Geometry: final body of the model. Coordinates: model frame, mm. A direction names the side the tool comes from. Coordinates: 2 decimals unless noted, no trailing zeros. Order: outer loops, then holes, each group sorted by start corner. A loop starts at its lowest first (then second) coordinate and runs counter-clockwise, first axis right, second up. Notation, with made-up numbers: M -20,84 L -2,84 A28 cw -2,107 Z; hole C -17,76 d5. An arc over 180 degrees is marked long. One line per question, with ' | ' between items.
Autodesk Inventor part; units mm, degrees
ref_plane "YZ Plane" through (0, 0, 0) normal (1, 0, 0) x (0, 1, 0)
ref_plane "XZ Plane" through (0, 0, 0) normal (0, 1, 0) x (-1, 0, 0)
ref_plane "XY Plane" through (0, 0, 0) normal (0, 0, 1) x (1, 0, 0)
sketch "Boceto1" plane through (0, 0, 0) normal (0, 1, 0) x (-1, 0, 0)
  line L0 (-14.8958, 23.7803) -> (7.8042, 23.7803)
  line L1 (7.8042, 23.7803) -> (7.8042, -7.6197)
  line L2 (7.8042, -7.6197) -> (-14.8958, -7.6197)
  line L3 (-14.8958, -7.6197) -> (-14.8958, 23.7803)
  line L4 (-14.8958, 23.7803) -> (7.8042, -7.6197) construction
  line L5 (7.8042, 23.7803) -> (-14.8958, -7.6197) construction
  arc A0 (-14.8958, 23.7803) -> (-14.8958, -7.6197) centre (0.5156, 8.0803) ccw
  line L6 (7.8042, 17.8112) -> (7.8042, 23.7803)
  line L7 (-13.6958, 20.5803) -> (6.6042, 20.5803)
  line L8 (6.6042, 20.5803) -> (6.6042, -4.4197)
  line L9 (6.6042, -4.4197) -> (-13.6958, -4.4197)
  line L10 (-13.6958, -4.4197) -> (-13.6958, 20.5803)
  line L11 (-13.6958, 20.5803) -> (6.6042, -4.4197) construction
  line L12 (6.6042, 20.5803) -> (-13.6958, -4.4197) construction
  line L13 (7.8042, 23.7803) -> (11.6042, 23.7803)
  line L14 (11.6042, 23.7803) -> (11.6042, -7.6197)
  line L15 (11.6042, -7.6197) -> (7.8042, -7.6197)
  line L16 (7.8042, -7.6197) -> (7.8042, 23.7803)
  line L17 (7.8042, 23.7803) -> (6.6042, 23.7803)
  line L18 (6.6042, 23.7803) -> (6.6042, -7.6197)
  line L19 (6.6042, -7.6197) -> (7.8042, -7.6197)
  line L20 (7.8042, -7.6197) -> (7.8042, 23.7803)
  line L21 (11.6042, -7.6197) -> (6.6042, -7.6197)
  line L22 (6.6042, -7.6197) -> (6.6042, -4.4197)
  line L23 (6.6042, -4.4197) -> (11.6042, -4.4197)
  line L24 (11.6042, -4.4197) -> (11.6042, -7.6197)
  line L25 (11.6042, 23.7803) -> (6.6042, 23.7803)
  line L26 (6.6042, 23.7803) -> (6.6042, 20.5803)
  line L27 (6.6042, 20.5803) -> (11.6042, 20.5803)
  line L28 (11.6042, 20.5803) -> (11.6042, 23.7803)
  line L29 (-14.8958, 23.7803) -> (-13.6958, 23.7803)
  line L30 (-13.6958, 23.7803) -> (-13.6958, -7.6197)
  line L31 (-13.6958, -7.6197) -> (-14.8958, -7.6197)
  line L32 (-14.8958, -7.6197) -> (-14.8958, 23.7803)
  point P0 (-3.5458, 8.0803)
  point P1 (6.6042, -4.4197)
  point P2 (6.6042, 20.5803)
  point P3 (6.6042, 23.7803)
  point P4 (6.6042, 20.5803)
  point P5 (11.6042, -4.4197)
  point P6 (6.6042, -4.4197)
  dimension "d4" = 25
  dimension "d5" = 3.2
  dimension "d6" = 1.2
  dimension "d7" = 20.3
  dimension "d14" = 5
  dimension "d34" = 22
extrude "Extrusión1" add sketch "Boceto1" along normal blind 12 contours L0 L30 L10 L2 L3 | L3 A0
sketch "Boceto3" plane through (0, 0, 0) normal (0, -1, 0) x (1, 0, 0)
  line L0 (10.8958, -4.4197) -> (16.4958, -4.4197)
  line L1 (16.4958, -4.4197) -> (16.4958, 20.5803)
  line L2 (16.4958, 20.5803) -> (10.8958, 20.5803)
  line L3 (10.8958, 20.5803) -> (10.8958, -4.4197)
  line L4 (13.6958, -7.6197) -> (13.6958, 23.7803)
  line L5 (10.8958, -4.4197) -> (16.4958, 20.5803) construction
  line L6 (16.4958, -4.4197) -> (10.8958, 20.5803) construction
  point P0 (0, 0)
  point P1 (13.6958, 8.0803)
  point P2 (13.6958, 20.5803)
  point P3 (13.6958, -4.4197)
  dimension "d18" = 25
  dimension "d19" = 2.8
extrude "Extrusión3" add sketch "Boceto3" along normal blind 15 contours L4 L2 L1 L0
fillet "Empalme2" radius 2 9 edges at (15.0958, 0, 20.5803) (15.0958, -15, 20.5803) (15.0958, -15, -4.4197) (15.0958, 0, -4.4197) (14.2958, 0, -7.6197) (14.2958, 12, -7.6197) (14.2958, 0, 23.7803) (14.2958, 12, 23.7803) (16.4958, 0, 8.0803)
sketch "Boceto4" plane through (16.4958, -13, -4.4197) normal (1, 0, 0) x (0, 0, -1)
  circle A0 centre (-19.5, 2.7) radius 2.7
  circle A1 centre (-5.5, 2.7) radius 2.7
  line L0 (-19.5, 5.4) -> (-5.5, 5.4)
  line L1 (-5.5, 5.4) -> (-5.5, 0)
  line L2 (-5.5, 0) -> (-19.5, 0)
  line L3 (-19.5, 0) -> (-19.5, 5.4)
  line L4 (-25, 11) -> (-25, 0)
  line L5 (0, 11) -> (0, 0)
  line L6 (-2, -2) -> (-23, -2)
  point P0 (-4.4197, 13)
  point P1 (-5.5, 0)
  point P2 (-5.5, 5.4)
  point P3 (-19.5, 5.4)
  dimension "d23" = 5.4
  dimension "d24" = 5.5
  dimension "d25" = 5.5
  dimension "d26" = 2
extrude "Extrusión4" cut sketch "Boceto4" against normal through all
sketch "Boceto5" plane through (16.4958, -13, -4.4197) normal (1, 0, 0) x (0, 0, -1)
  arc A0 (-5.5, 0) -> (-5.5, 5.4) centre (-5.5, 2.7) ccw
  line L0 (-5.5, 0) -> (-19.5, 0)
  arc A1 (-19.5, 5.4) -> (-19.5, 0) centre (-19.5, 2.7) ccw
  line L1 (-19.5, 5.4) -> (-5.5, 5.4)
  arc A2 (-2, -2) -> (0, 0) centre (-2, 0) ccw
  line L2 (0, 11) -> (0, 0)
  line L3 (-25, 11) -> (0, 11)
  line L4 (-25, 11) -> (-25, 0)
  arc A3 (-25, 0) -> (-23, -2) centre (-23, 0) ccw
  line L5 (-2, -2) -> (-23, -2)
  arc A4 (-5.5, -2) -> (-5.5, 7.4) centre (-5.5, 2.7) ccw
  line L6 (-5.5, -2) -> (-19.5, -2)
  arc A5 (-19.5, 7.4) -> (-19.5, -2) centre (-19.5, 2.7) ccw
  line L7 (-19.5, 7.4) -> (-5.5, 7.4)
  point P0 (-4.4197, 13)
  point P1 (-21.3974, 7)
  point P2 (-19.5, -2)
  point P3 (-5.5, -2)
  point P4 (-3.6026, 7)
  dimension "d29" = 2
sketch "Boceto2" plane through (-6.6042, 0, 23.7803) normal (0, 0, 1) x (1, 0, 0)
  circle A0 centre (2.3, 6) radius 2.7
  line L0 (-5, 0) -> (21.5, 0)
  circle A1 centre (10.3, 6) radius 2.7
  line L1 (2.3, 3.3) -> (10.3, 3.3)
  line L2 (10.3, 3.3) -> (10.3, 8.7)
  line L3 (10.3, 8.7) -> (2.3, 8.7)
  line L4 (2.3, 8.7) -> (2.3, 3.3)
  point P0 (6.6042, 0)
  point P1 (20.3, 0)
  dimension "d10" = 5.4
  dimension "d11" = 6
  dimension "d12" = 10
  dimension "d13" = 8
properties part number "yystop"
1. Section D-D, the plane z = 11. Output: boundary loops of the cut face in (x, y).
Response values:
outline: M 13.7,-15 L 16.5,-15 L 16.5,-13 L 13.7,-13 Z; M 13.7,-7.6 L 16.5,-7.6 L 16.5,-2 A2 cw 18.5,0 L 21.29,0 L 21.29,12 L 13.7,12 Z
2. Section B-B, the plane z = -0.5. Output: boundary loops of the cut face in (x, y), and give its area (3 significant figures).
Response values:
outline: M 13.7,-15 L 16.5,-15 L 16.5,-12.49 L 13.7,-12.49 Z; M 13.7,-8.11 L 16.5,-8.11 L 16.5,-2 A2 cw 18.5,0 L 19.74,0 L 19.74,12 L 13.7,12 Z | area: 103 mm^2
3. Draft query along Z for faces 6 (the face through (16.496, -7, 8)), 7 (the face through (15, -7.6, 8)), 8 (the face through (21.483, 5.644, 7.836)). Return one class per face: pulls with the +Z half, pulls with the -Z half, needs draft (parallel to the pull), parting line crosses it, or undercut.
Response values:
face 6: needs draft | face 7: undercut | face 8: parting line crosses it
4. Material intervals for line 1 (Z direction, x = 15.5, y = -10.5); line 2 (Y direction, x = 14, z = 15); line 3 (Y direction, x = 19, z = 6), sorted ascending. Write a range as [from, to].
Response values:
line 1: z = [-4.42, -1.61], [17.77, 20.58] | line 2: y = [-15, -13], [-7.6, 12] | line 3: y = [0, 12]
5. Access query for faces 1 (the face through (20, 0, 8)), 2 (the face through (15, -7, -4.42)), 3 (the face through (15.12, -14.4, 20.01)), 4 (the face through (15, -13, 8)), 5 (the face through (15, -15, 8)). Directions: +Z, -Z, +X, -X, +Y, -Y. A direction counts if a zero-diameter tool reaches every point of the face in a straight line with its end or side. Return the directions, or none.
Response values:
face 1: +Z, -Z, +X, -Y | face 2: -Z, +X, -X, -Y | face 3: +Z, +X, -X, -Y | face 4: +X, -X | face 5: +Z, -Z, +X, -X, -Y
6. Pin query (flat end, axial travel): P1, Ø10, axis at y = -9, z = 11, coming from the +X side; P2, Ø3.5, axis at x = 19.5, z = 10.5, coming from the -Y side; P3, Ø3, axis at x = 15, y = -7, coming from the -Z side; P4, Ø1, axis at x = 18, y = -5, coming from the +Z side. Return the tip coordinate at first contact, or that it passes through.
Response values:
P1: stops at x = 16.5 | P2: stops at y = -0.14 | P3: stops at z = -4.42 | P4: passes through
7. Section C-C, the plane x = 16. Output: boundary loops of the cut face in (y, z), and give its area (3 significant figures).
Response values:
outline: M -15,-2.42 A2 ccw -13,-4.42 L -2,-4.42 A2 cw -0.04,-6.02 A2 ccw 0.1,-6.45 L 11.82,-6.45 A2 ccw 12,-5.62 L 12,21.78 A2 ccw 11.82,22.61 L 0.1,22.61 A2 ccw -0.04,22.18 A2 cw -2,20.58 L -13,20.58 A2 ccw -15,18.58 Z; hole M -13,1.08 A2.7 ccw -7.6,1.08 L -7.6,15.08 A2.7 ccw -13,15.08 Z | area: 625 mm^2
8. Section A-A, the plane y = -10.3. Output: boundary loops of the cut face in (x, z), and give its area (3 significant figures).
Response values:
outline: M 13.7,-4.42 L 16.5,-4.42 L 16.5,-1.62 L 13.7,-1.62 Z; M 13.7,17.78 L 16.5,17.78 L 16.5,20.58 L 13.7,20.58 Z | area: 15.7 mm^2
